Autodesk Inventor part; units mm, degrees
ref_plane "YZ Plane" through (0, 0, 0) normal (1, 0, 0) x (0, 1, 0)
ref_plane "XZ Plane" through (0, 0, 0) normal (0, 1, 0) x (-1, 0, 0)
ref_plane "XY Plane" through (0, 0, 0) normal (0, 0, 1) x (1, 0, 0)
sketch "Boceto1" plane through (0, 0, 0) normal (0, 1, 0) x (-1, 0, 0)
  arc A0 (-10.02, 7.27) -> (-8.75, 6) centre (-8.75, 7.27) ccw
  line L0 (-8.75, 6) -> (-2.54, 6)
  arc A1 (-1.27, 4.73) -> (-2.54, 6) centre (-2.54, 4.73) ccw
  line L1 (-1.27, 4.73) -> (-1.27, 1.27)
  arc A2 (-1.27, 1.27) -> (0, 0) centre (0, 1.27) ccw
  line L2 (0, 0) -> (62.46, 0)
  arc A3 (62.46, 0) -> (63.73, 1.27) centre (62.46, 1.27) ccw
  line L3 (63.73, 1.27) -> (63.73, 4.73)
  arc A4 (65, 6) -> (63.73, 4.73) centre (65, 4.73) ccw
  line L4 (65, 6) -> (71.21, 6)
  arc A5 (71.21, 6) -> (72.48, 7.27) centre (71.21, 7.27) ccw
  line L5 (72.48, 7.27) -> (72.48, 21.73)
  arc A6 (72.48, 21.73) -> (71.21, 23) centre (71.21, 21.73) ccw
  line L6 (71.21, 23) -> (65, 23)
  arc A7 (63.73, 24.27) -> (65, 23) centre (65, 24.27) ccw
  line L7 (63.73, 24.27) -> (63.73, 27.73)
  arc A8 (63.73, 27.73) -> (62.46, 29) centre (62.46, 27.73) ccw
  line L8 (62.46, 29) -> (0, 29)
  arc A9 (0, 29) -> (-1.27, 27.73) centre (0, 27.73) ccw
  line L9 (-1.27, 27.73) -> (-1.27, 24.27)
  arc A10 (-2.54, 23) -> (-1.27, 24.27) centre (-2.54, 24.27) ccw
  line L10 (-2.54, 23) -> (-8.75, 23)
  arc A11 (-8.75, 23) -> (-10.02, 21.73) centre (-8.75, 21.73) ccw
  line L11 (-10.02, 21.73) -> (-10.02, 7.27)
  circle A12 centre (61.755, 25.475) radius 1.25
  circle A13 centre (0.755, 3.475) radius 1.25
  circle A14 centre (0.755, 25.475) radius 1.25
  circle A15 centre (61.755, 3.475) radius 1.25
  circle A16 centre (38.98, 14.5) radius 0.9
  circle A17 centre (23.98, 14.5) radius 0.9
  point P0 (0, 0)
extrude "Extrusión1" add sketch "Boceto1" along normal blind 1.04
sketch "Boceto2" plane through (0, 1.04, 0) normal (0, 1, 0) x (1, 0, 0)
  circle A0 centre (-65.48, -14.5) radius 0.9
  circle A1 centre (3.02, -14.5) radius 0.9
  line L0 (-71.21, -23) -> (-65, -23)
  line L1 (-72.48, -7.27) -> (-72.48, -21.73)
  line L2 (2.54, -23) -> (8.75, -23)
  line L3 (10.02, -21.73) -> (10.02, -7.27)
  point P0 (0, 0)
  dimension "d2" = 1.8
  dimension "d3" = 1.8
  dimension "d4" = 8.5
  dimension "d5" = 7
  dimension "d6" = 8.5
  dimension "d7" = 7
hole "Agujero1" at (-65.48, 1.04, 14.5) at (3.02, 1.04, 14.5) direction (0, -1, 0) diameter 1.8 end through all
sketch "Boceto3" plane through (0, 1.04, 0) normal (0, 1, 0) x (1, 0, 0)
  circle A0 centre (-3.08, -11.96) radius 0.4
  line L0 (0, 0) -> (-62.46, 0)
  line L1 (10.02, -21.73) -> (10.02, -7.27)
  circle A1 centre (-3.08, -14.5) radius 0.4
  circle A2 centre (-3.08, -17.04) radius 0.4
  line L2 (-62.46, -29) -> (0, -29)
  line L3 (1.27, -27.73) -> (1.27, -24.27)
  dimension "d23" = 0.8
  dimension "d24" = 11.96
  dimension "d25" = 13.1
  dimension "d26" = 0.8
  dimension "d27" = 0.8
  dimension "d28" = 13.1
  dimension "d29" = 13.1
  dimension "d30" = 11.96
  dimension "d31" = 2.54
  dimension "d32" = 2.54
  dimension "d40" = 4.35
hole "Agujero2" at (-3.08, 1.04, 11.96) at (-3.08, 1.04, 14.5) at (-3.08, 1.04, 17.04) direction (0, -1, 0) diameter 0.8 end through all
sketch "Boceto4" plane through (0, 0, 0) normal (0, -1, 0) x (1, 0, 0)
  line L0 (4.72, 9.6) -> (1.32, 9.6)
  line L1 (1.32, 9.6) -> (1.32, 12)
  line L2 (1.32, 12) -> (4.72, 12)
  line L3 (4.72, 12) -> (4.72, 9.6)
  line L4 (4.72, 17) -> (1.32, 17)
  line L5 (1.32, 17) -> (1.32, 19.4)
  line L6 (1.32, 19.4) -> (4.72, 19.4)
  line L7 (4.72, 19.4) -> (4.72, 17)
  line L8 (10.02, 21.73) -> (10.02, 7.27)
  line L9 (2.54, 23) -> (8.75, 23)
  line L10 (8.75, 6) -> (2.54, 6)
  line L11 (-63.78, 19.4) -> (-67.18, 19.4)
  line L12 (-67.18, 19.4) -> (-67.18, 17)
  line L13 (-67.18, 17) -> (-63.78, 17)
  line L14 (-63.78, 17) -> (-63.78, 19.4)
  line L15 (-71.21, 23) -> (-65, 23)
  line L16 (-72.48, 7.27) -> (-72.48, 21.73)
  line L17 (-63.78, 9.6) -> (-67.18, 9.6)
  line L18 (-67.18, 9.6) -> (-67.18, 12)
  line L19 (-67.18, 12) -> (-63.78, 12)
  line L20 (-63.78, 12) -> (-63.78, 9.6)
  line L21 (-65, 6) -> (-71.21, 6)
  point P0 (0, 0)
  dimension "d41" = 3.4
  dimension "d42" = 2.4
  dimension "d43" = 3.4
  dimension "d44" = 2.4
  dimension "d45" = 5.3
  dimension "d46" = 3.6
  dimension "d47" = 3.6
  dimension "d48" = 3.4
  dimension "d49" = 2.4
  dimension "d50" = 3.6
  dimension "d51" = 5.3
  dimension "d52" = 3.6
  dimension "d53" = 5.3
extrude "Extrusión2" cut sketch "Boceto4" against normal through all
properties part number "Interstage B1"
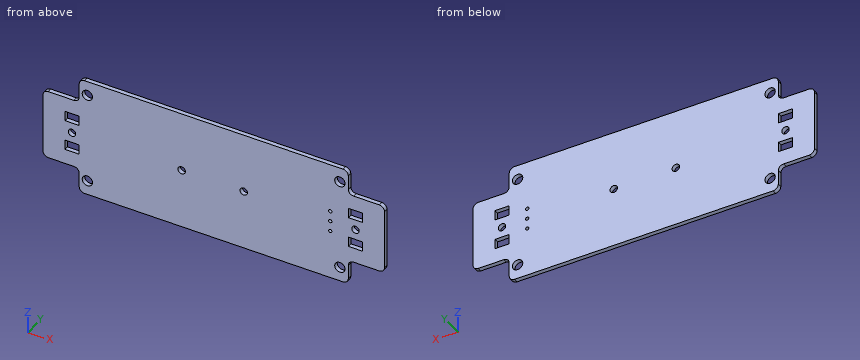
CAD build for the part. Positions are in the model's coordinates, mm. Give positions to 0.01 mm unless a question says otherwise; leave off trailing zeros. Write each loop counter-clockwise with the first axis right and the second up, starting at its lowest first coordinate (ties: lowest second). Pieces come first, ordered by that corner, then holes. Notation, with made-up numbers: M 68.25,15 L 122.25,15 A25 cw 122.25,41 Z; hole C 69,-19 d6. An arc over 180 degrees is marked long. Return JSON: item names as keys, results as strings. Group by question number.
(1) Band-saw the part on C-C (y = 0.3). State how many separate pieces and enclosed holes the cut face has, and give its area (3 significant figures).
(2) Flat gauge pin, fed straight in: pin 1 Ø0.5 at (x, y) = (-66.5, 0.5) entering from -Z. Where does the tip first touch, or does it go through?
(3) Band-saw the part on A-A (z = 18.25). Give the cut face in (x, y).
(4) Drill centre lines: L1, parallel to Z at x = -3.08, y = 0.55; L2, parallel to X at y = 0.85, z = 19; L3, parallel to Z at x = -67, y = 0.9. Where is each one in solid material? Low to high. Write a range as [from, to].
(5) Band-saw the part on B-B (x = -23.98). Give the cut face in (y, z).
Entries:
{
 "1": {"separate pieces": "1", "enclosed holes": "15", "area": "2,120 mm^2"},
 "2": {"pin 1": "stops at z = 6"},
 "3": {"outline": "M -72.48,0 L -67.18,0 L -67.18,1.04 L -72.48,1.04 Z; M -63.78,0 L 1.32,0 L 1.32,1.04 L -63.78,1.04 Z; M 4.72,0 L 10.02,0 L 10.02,1.04 L 4.72,1.04 Z"},
 "4": {"L1": "z = [0, 11.56], [12.36, 14.1], [14.9, 16.64], [17.44, 29]", "L2": "x = [-72.48, -67.18], [-63.78, 1.32], [4.72, 10.02]", "L3": "z = [6, 9.6], [12, 17], [19.4, 23]"},
 "5": {"outline": "M 0,0 L 1.04,0 L 1.04,13.6 L 0,13.6 Z; M 0,15.4 L 1.04,15.4 L 1.04,29 L 0,29 Z"}
}
